from build123d import *

# Parameters (mm, degrees)
HUB_DIAMETER_R      = 61
HUB_DEPTH           = 24
FLANGE_DIAMETER_R   = 90
FLANGE_DEPTH        = 21
SKETCH_1_R          = 38
CUT_EXTRUDE_1_DEPTH = 130.52219887


with BuildPart() as part:
    # Hub Diameter → Hub (new body)
    with BuildSketch(Plane.XY):
        Circle(HUB_DIAMETER_R)
    extrude(amount=-HUB_DEPTH)

    # Flange Diameter → Flange (add)
    with BuildSketch(Plane.XY.offset(-3)):
        Circle(FLANGE_DIAMETER_R)
    extrude(amount=-FLANGE_DEPTH)

    # Эскиз1 → Вырез-Вытянуть1 (cut, through all)
    with BuildSketch(Plane.XY):
        Circle(SKETCH_1_R)
    extrude(amount=-CUT_EXTRUDE_1_DEPTH, mode=Mode.SUBTRACT)


solid = part.part
Geometry check sheet. Reference: the model listing, model coordinates, mm. A direction names the side the tool comes from. Round coordinates to 2 decimals unless told otherwise and drop trailing zeros. Loops run counter-clockwise (first coordinate to the right, second up) from the corner with the lowest first, then second, coordinate; pieces in that order, holes last.
Item 1: Gauge pin test, flat ends, axial feed: pin 1 (4 mm diameter, centred on y = -32, z = -15.5, fed in from +X); pin 2 (3 mm diameter, centred on x = -28, z = -5.5, fed in from -Y); pin 3 (8 mm diameter, centred on x = -61, z = -3.5, fed in from -Y); pin 4 (4 mm diameter, centred on x = 38.5, y = -27, fed in from +Z). Record the tip position at first contact, or that the pin passes through.
Item 2: Cross-section at C-C on x = -51. Record the boundary of the cut face in (y, z).
Item 3: Access from +Z, -Z, +X, -X, +Y, -Y to the whole of each face (thin tool, end or side, straight path). Record for faces 4 (the flat face through (-28, -26, 0)), 5 (the cylindrical face through (-48.408, -37.118, -1.479)).
Item 4: Cross-section at D-D on z = -8.25. Record the boundary of the cut face in (x, y), then the cut area to 3 significant figures.
Item 5: Mould release check, pull along X, two halves, no side actions. Record for faces 1 (the flat face through (39, 1, -24)), 2 (the cylindrical face through (41.53, -79.845, -13.353)), 3 (the cylindrical face through (17.535, -33.713, -11.832)): pulls with the +X half, pulls with the -X half, needs draft (parallel to the pull), parting line crosses it, or undercut.
Item 6: Cross-section at A-A on y = 0. Record the boundary of the cut face in (x, z).
Item 7: Thickness scan on line 1 (Y direction, x = 0, z = -8.5); line 2 (X direction, y = 1, z = -15.75); line 3 (Z direction, x = -70.5, y = 43). Record the ranges inside material, lowest first.
Answer sheet:
1. pin 1: stops at x = 84.85
1. pin 2: stops at y = -86.01
1. pin 3: stops at y = -69.65
1. pin 4: stops at z = 0
2. outline: (-74.16, -24) - (74.16, -24) - (74.16, -3) - (33.47, -3) - (33.47, 0) - (-33.47, 0) - (-33.47, -3) - (-74.16, -3) - close
3. face 4: +Z, +X, -X, +Y, -Y
3. face 5: +Z
4. outline: circle Ø180 at (0, 0); hole circle Ø76 at (0, 0)
4. area: 20,900 mm2
5. face 1: needs draft
5. face 2: parting line crosses it
5. face 3: undercut
6. outline: (-90, -24) - (-38, -24) - (-38, 0) - (-61, 0) - (-61, -3) - (-90, -3) - close; (38, -24) - (90, -24) - (90, -3) - (61, -3) - (61, 0) - (38, 0) - close
7. line 1: y = -90 to -38, 38 to 90
7. line 2: x = -89.99 to -37.99, 37.99 to 89.99
7. line 3: z = -24 to -3
